Autodesk Inventor part; units mm, degrees
ref_plane "YZ Plane" through (0, 0, 0) normal (1, 0, 0) x (0, 1, 0)
ref_plane "XZ Plane" through (0, 0, 0) normal (0, 1, 0) x (-1, 0, 0)
ref_plane "XY Plane" through (0, 0, 0) normal (0, 0, 1) x (1, 0, 0)
sketch "スケッチ1" plane through (0, 0, 0) normal (0, 0, 1) x (1, 0, 0)
  line L0 (5, -5) -> (-5, -5)
  line L1 (-5, -5) -> (-5, 5)
  line L2 (-5, 5) -> (5, 5)
  line L3 (5, 5) -> (5, -5)
  line L4 (5, -5) -> (-5, 5) construction
  line L5 (-5, -5) -> (5, 5) construction
  line L6 (4, 4) -> (-4, 4)
  line L7 (-4, 4) -> (-4, -4)
  line L8 (-4, -4) -> (4, -4)
  line L9 (4, -4) -> (4, 4)
  point P0 (0, 0)
  dimension "d0" = 10
  dimension "d1" = 10
  dimension "d2" = 1
extrude "押し出し1" add sketch "スケッチ1" along normal blind 90
sketch "スケッチ2" plane through (5, -5, 0) normal (1, 0, 0) x (0, 0, -1)
  line L0 (0, 0) -> (0, 10)
  line L1 (0, 10) -> (-90, 10)
  line L2 (-90, 0) -> (-90, 10)
  line L3 (0, 0) -> (-90, 0)
  line L4 (-90, 5) -> (0, 5)
  point P0 (-50, 5)
  point P1 (-5, 5)
  dimension "d5" = 45
  dimension "d6" = 5
hole "穴1" at (5, 0, 50) at (5, 0, 5) direction (-1, 0, 0) diameter 3.3 end through all
sketch "スケッチ3" plane through (-5, 5, 0) normal (0, 1, 0) x (1, 0, 0)
  line L0 (10, 0) -> (0, 0)
  line L1 (0, 0) -> (0, -90)
  line L2 (10, -90) -> (0, -90)
  line L3 (10, 0) -> (10, -90)
  line L4 (5, -90) -> (5, 0)
  point P0 (5, -60)
  point P1 (5, -10)
  dimension "d14" = 50
  dimension "d15" = 10
hole "穴2" at (0, 5, 60) at (0, 5, 10) direction (0, -1, 0) diameter 3.3 end through all
properties part number "kaku_1010_120"
The model under review builds one solid part; all positions refer to its coordinate system, in mm. A direction names the side the tool comes from. Round coordinates to 2 decimals unless told otherwise and drop trailing zeros. Order: outer loops, then holes, each group sorted by start corner. A loop starts at its lowest first (then second) coordinate and runs counter-clockwise, first axis right, second up. Notation, with made-up numbers: M 28,26 L 40,26 A30 cw 40,51 Z; hole C 37,-33 d9. An arc over 180 degrees is marked long. Use a Markdown table: item, result.
1) Consider section B-B (y = -2.5). Write out the cut boundary in (x, z), then the cut area to 3 significant figures.
Report:
| item | result |
|---|---|
| outline | M -5,0 L -4,0 L -4,90 L -5,90 Z; M 4,0 L 5,0 L 5,90 L 4,90 Z |
| area | 180 mm^2 |
2) Consider section A-A (z = 5). Write out the cut boundary in (x, y), then the cut area to 3 significant figures.
Report:
| item | result |
|---|---|
| outline | M -5,-5 L 5,-5 L 5,-1.65 L 4,-1.65 L 4,-4 L -4,-4 L -4,-1.65 L -5,-1.65 Z; M -5,1.65 L -4,1.65 L -4,4 L 4,4 L 4,1.65 L 5,1.65 L 5,5 L -5,5 Z |
| area | 29.4 mm^2 |
3) Wall thickness on line 1 along Z through (x, y) = (0, 4.75); line 2 along Z through (x, y) = (-4.2, 0); line 3 along Y through (x, z) = (-2, 47): over which ranges is each line inside the solid? List them lowest first. Write a range as [from, to].
Report:
| item | result |
|---|---|
| line 1 | [0, 8.35], [11.65, 58.35], [61.65, 90] |
| line 2 | [0, 3.35], [6.65, 48.35], [51.65, 90] |
| line 3 | [-5, -4], [4, 5] |
4) Tool access review of faces 4 (the face through (-4, 0, 44)), 5 (the face through (-4.51, -0.07, 6.65)): name each direction out of +Z, -Z, +X, -X, +Y, -Y from which nothing blocks a thin tool from reaching the whole face with its end or side.
Report:
| item | result |
|---|---|
| face 4 | +Z, -Z |
| face 5 | +X, -X |
5) Draft analysis for pull direction Z (two halves, no side actions). For faces 1 (the face through (4.49, -0.07, 51.65)), 2 (the face through (-4.5, 0.1, 0)), 3 (the face through (-5, 0, 44)), state which applies: released by +Z, released by -Z, zero draft, split by the parting line, or undercut.
Report:
| item | result |
|---|---|
| face 1 | undercut |
| face 2 | released by -Z |
| face 3 | zero draft |
6) Consider section C-C (z = 67). Write out the cut boundary in (x, y), then the cut area to 3 significant figures.
Report:
| item | result |
|---|---|
| outline | M -5,-5 L 5,-5 L 5,5 L -5,5 Z; hole M -4,-4 L 4,-4 L 4,4 L -4,4 Z |
| area | 36.0 mm^2 |
